Check sheet for the modelled part. Datum: model origin and axes. Units: mm. Give positions to 0.01 mm unless a question says otherwise; leave off trailing zeros. Loops run counter-clockwise (first coordinate to the right, second up) from the corner with the lowest first, then second, coordinate; pieces in that order, holes last. Notation, with made-up numbers: (20, 76.5) - (77, 76.5) arc R30 cw to (77, 101.5) - close; hole circle Ø3 at (59.5, 38.5). An arc over 180 degrees is marked (long way). Use one line per item in the form item = value.
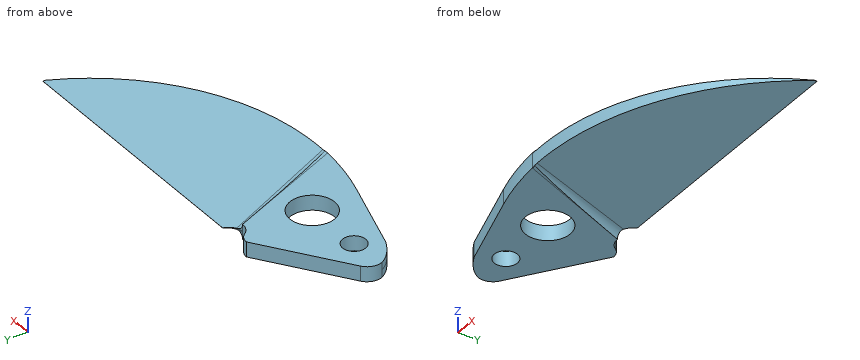
from build123d import *

# Parameters (mm, degrees)
SCHIZZO1_R                   = 3
ESTRUSIONE_ESTRUSIONE1_DEPTH = 1
ESTRUSIONE_ESTRUSIONE2_DEPTH = 0.95
SMUSSO1_SIZE                 = 18
SMUSSO1_SIZE_2               = 0.943340027
SMUSSO2_SIZE                 = 18
SMUSSO2_SIZE_2               = 0.943340027
RACCORDO1_R                  = 0.9
RACCORDO2_R                  = 0.9
TAGLIO_ESTRUSIONE1_DEPTH     = 10
RACCORDO3_R                  = 2
SCHIZZO3_R                   = 1.55
TAGLIO_ESTRUSIONE2_DEPTH     = 41.278810137


with BuildPart() as part:
    # Schizzo1 → Estrusione-Estrusione1 (new, symmetric)
    with BuildSketch(Plane.XY):
        with BuildLine():
            Line((-0.88, 9.5), (-19.130944839, 9.5))
            ThreePointArc((-19.130944839, 9.5), (-20.501263026, 8.610104965), (-20.245662077, 6.99630409))
            Line((-20.245662077, 6.99630409), (-15.960328698, 2.236959209))
            Line((-15.960328698, 2.236959209), (-14.839064722, 1.115695234))
            ThreePointArc((-14.839064722, 1.115695234), (-14.577677448, 0.895591951), (-14.282636649, 0.723197957))
            ThreePointArc((-14.282636649, 0.723197957), (-13.491665822, 0.254040408), (-12.8, -0.352047083))
            add(Edge.make_bspline(
                [(-9.8, -3.018897494), (-12.016366306, -1.919392636), (-12.8, -0.352047083)],
                knots=[0, 0, 0, 0.799118898, 0.799118898, 0.799118898], degree=2))
            Line((-9.8, -3.018897494), (0.594713885, -6.396344771))
            ThreePointArc((0.594713885, -6.396344771), (4.37641373, -7.379985604), (8.248348818, -7.906219091))
            Line((8.248348818, -7.906219091), (2.2, 7.850268275))
            ThreePointArc((2.2, 7.850268275), (1.255676497, 8.087244418), (0.535135135, 8.742015153))
            ThreePointArc((0.535135135, 8.742015153), (-0.077325022, 9.298570279), (-0.88, 9.5))
        make_face()
        Circle(SCHIZZO1_R, mode=Mode.SUBTRACT)
    extrude(amount=ESTRUSIONE_ESTRUSIONE1_DEPTH, both=True)

    # Schizzo1<4> → Estrusione-Estrusione2 (add, symmetric)
    with BuildSketch(Plane.XY):
        with BuildLine():
            ThreePointArc((4.091335816, 9.2), (3.361779551, 8.222303818), (2.2, 7.850268275))
            Line((2.2, 7.850268275), (8.248348818, -7.906219091))
            ThreePointArc((8.248348818, -7.906219091), (26.021901415, -4.20199667), (39.091335816, 8.4))
            Line((39.091335816, 8.4), (39.091335816, 8.7))
            Line((39.091335816, 8.7), (4.091335816, 9.2))
        make_face()
    extrude(amount=ESTRUSIONE_ESTRUSIONE2_DEPTH, both=True)

    # Smusso1
    # the kernel refuses this chamfer: 18, 0.943340027 mm, written as the material it takes off along each edge
    with BuildSketch(Plane(origin=(85.88418926, 8.031530665, 0.95), x_dir=(-0.01428422784103612, -0.9998959488725246, 0.002013023422382226), z_dir=(-0.99989797479951, 0.014284256782850195, 0))) as smusso1_piece_1_section:
        Polygon((SMUSSO1_SIZE * 0.999997973866, -SMUSSO1_SIZE * 0.00201302342238), (-SMUSSO1_SIZE_2 * 0.00201302342258, -SMUSSO1_SIZE_2 * 0.999997973967), (0, 0), align=None)
    smusso1_piece_1 = extrude(amount=128.598827208, mode=Mode.PRIVATE)
    smusso1_piece_1 = split(smusso1_piece_1, bisect_by=Plane(origin=(5.771356931, -1.453434613, 0.613202149), z_dir=(0.9335804264972009, 0.3583679495453028, 0)), keep=Keep.TOP, mode=Mode.PRIVATE)
    add(smusso1_piece_1, mode=Mode.SUBTRACT)

    # Smusso2
    # the kernel refuses this chamfer: 18, 0.943340027 mm, written as the material it takes off along each edge
    with BuildSketch(Plane(origin=(85.88418926, 8.031530665, -0.95), x_dir=(-0.01428422784103612, -0.9998959488725246, -0.002013023422382226), z_dir=(-0.99989797479951, 0.014284256782850195, 0))) as smusso2_piece_1_section:
        Polygon((SMUSSO2_SIZE * 0.999997973866, SMUSSO2_SIZE * 0.00201302342238), (-SMUSSO2_SIZE_2 * 0.00201302342258, SMUSSO2_SIZE_2 * 0.999997973967), (0, 0), align=None)
    smusso2_piece_1 = extrude(amount=128.598827208, mode=Mode.PRIVATE)
    smusso2_piece_1 = split(smusso2_piece_1, bisect_by=Plane(origin=(5.771356931, -1.453434613, -0.613202149), z_dir=(0.9335804264972009, 0.3583679495453028, 0)), keep=Keep.TOP, mode=Mode.PRIVATE)
    add(smusso2_piece_1, mode=Mode.SUBTRACT)

    # Raccordo1
    # the kernel refuses this fillet: 0.9 mm, written as the material it adds along each edge
    with BuildSketch(Plane(origin=(1.410141131, 9.907920978, -0.028429649), x_dir=(-0.017415293659521727, 0.04536839107084769, 0.9988185103603132), z_dir=(0.35794454152552274, -0.9324774108955555, 0.048596124964905896))) as raccordo1_piece_1_section:
        with BuildLine():
            CenterArc((RACCORDO1_R * 0.980734011967, -RACCORDO1_R), RACCORDO1_R, 90, 88.885438442)
            Line((-RACCORDO1_R * 0.0190767888902, -RACCORDO1_R * 0.980548457933), (0, 0))
            Line((0, 0), (RACCORDO1_R * 0.980734011967, 0))
        make_face()
    raccordo1_piece_1 = extrude(amount=21.310749772, mode=Mode.PRIVATE)
    raccordo1_piece_1 = raccordo1_piece_1 & Plane(origin=(10.715020451, 24.750756137, 0.600477284), x_dir=(-0.30901699437494573, -0.9510565162951542, 0), z_dir=(0, 0, 1)) * Cylinder(32.75, 47, mode=Mode.PRIVATE)
    raccordo1_piece_1 = split(raccordo1_piece_1, bisect_by=Plane(origin=(5.151176086, 0.789201867, 1), z_dir=(0, 0, -1)), keep=Keep.TOP, mode=Mode.PRIVATE)
    raccordo1_piece_1 = raccordo1_piece_1 - Plane(origin=(2.2, 9.850268275, 0.600477284), x_dir=(0, -1, 0), z_dir=(0, 0, 1)) * Cylinder(2, 47, mode=Mode.PRIVATE)
    add(raccordo1_piece_1)

    # Raccordo2
    # the kernel refuses this fillet: 0.9 mm, written as the material it adds along each edge
    with BuildSketch(Plane(origin=(1.410141131, 9.907920978, 0.028429649), x_dir=(-0.017415293659511128, 0.04536839107085176, -0.9988185103603133), z_dir=(0.35794454152552274, -0.9324774108955555, -0.048596124964905896))) as raccordo2_piece_1_section:
        with BuildLine():
            CenterArc((RACCORDO2_R * 0.980734011967, RACCORDO2_R), RACCORDO2_R, 181.114561558, 88.885438442)
            Line((-RACCORDO2_R * 0.0190767888902, RACCORDO2_R * 0.980548457933), (0, 0))
            Line((0, 0), (RACCORDO2_R * 0.980734011967, 0))
        make_face()
    raccordo2_piece_1 = extrude(amount=21.310749772, mode=Mode.PRIVATE)
    raccordo2_piece_1 = split(raccordo2_piece_1, bisect_by=Plane(origin=(5.151178194, 0.789195879, -1), z_dir=(0, 0, 1)), keep=Keep.TOP, mode=Mode.PRIVATE)
    raccordo2_piece_1 = raccordo2_piece_1 & Plane(origin=(10.715020451, 24.750756137, -0.600477223), x_dir=(-0.3090169943750401, -0.9510565162951234, 0), z_dir=(0, 0, 1)) * Cylinder(32.75, 47, mode=Mode.PRIVATE)
    raccordo2_piece_1 = raccordo2_piece_1 - Plane(origin=(2.2, 9.850268275, -0.600477223), x_dir=(0, -1, 0), z_dir=(0, 0, 1)) * Cylinder(2, 47, mode=Mode.PRIVATE)
    add(raccordo2_piece_1)

    # Schizzo2 → Taglio-Estrusione1 (cut)
    with BuildSketch(Plane.XY.offset(1)):
        Polygon((-0.88, 9.5), (-30.88, -10.735255505), (-30.88, 9.5), align=None)
    extrude(amount=-TAGLIO_ESTRUSIONE1_DEPTH, mode=Mode.SUBTRACT)

    # Raccordo3
    # the kernel refuses this fillet: 2 mm, written as the material it takes off along each edge
    with BuildSketch(Plane(origin=(-14.059482684, 0.610326682, -7.107620692), x_dir=(0.7945891525397701, -0.6071474933375991, 0), z_dir=(0, 0, 1))) as raccordo3_piece_1:
        with BuildLine():
            CenterArc((2.675251835, 1.676756542), RACCORDO3_R, 161.383532721, 75.585730468)
            Line((0.779898436, 2.315219927), (0.741991368, 2.327989195))
            Line((0.741991368, 2.327989195), (-0.037907068, 0.012769268))
            Line((-0.037907068, 0.012769268), (0.006340296, -0.039494312))
            ThreePointArc((0.006340296, -0.039494312), (0.792537049, 0.023211061), (1.563270543, -0.033535131))
            Line((1.563270543, -0.033535131), (1.585074098, 0))
        make_face()
    extrude(amount=14.215241383, mode=Mode.SUBTRACT)

    # Schizzo3 → Taglio-Estrusione2 (cut, through all)
    with BuildSketch(Plane(origin=(0, 0, -1), x_dir=(-1, 0, 0), z_dir=(0, 0, -1))):
        with Locations((8, 0)):
            Circle(SCHIZZO3_R)
    extrude(amount=-TAGLIO_ESTRUSIONE2_DEPTH, mode=Mode.SUBTRACT)


solid = part.part
Item 1: Section check A-A on x = 0. Record the boundary of the cut face in (y, z), then the cut area to 3 significant figures.
Answer block:
outline = (-6.2, -1) - (-3, -1) - (-3, 1) - (-6.2, 1) - close; (3, -1) - (9.25, -1) - (9.25, 1) - (3, 1) - close
area = 18.9 mm2
Item 2: Section check B-B on y = 0.5. Give the number of separate pieces and of enclosed holes in the cut face, then the cut area to 3 significant figures.
Answer block:
separate_pieces = 3
enclosed_holes = 0
area = 43.5 mm2
Item 3: Gauge pin test, flat ends, axial feed: P1, Ø10, axis at x = 25.5, y = 7, coming from the +Z side; P2, Ø3, axis at x = -8, y = 0, coming from the +Z side. Record the tip position at first contact, or that the pin passes through.
Answer block:
P1 = 0.37
P2 = through
Item 4: Section check D-D on x = -8. Record the boundary of the cut face in (y, z).
Answer block:
outline = (-3.6, -1) - (-1.55, -1) - (-1.55, 1) - (-3.6, 1) - close; (1.55, -1) - (4.7, -1) - (4.7, 1) - (1.55, 1) - close
Item 5: Thickness scan on L1, parallel to X at y = -2, z = -0.4; L2, parallel to Y at x = -8, z = 0.55; L3, parallel to Y at x = -0.5, z = 0.55. Record the ranges inside material, lowest first.
Answer block:
L1 = -11.42 to -2.24, 2.24 to 29.61
L2 = -3.6 to -1.55, 1.55 to 4.7
L3 = -6.04 to -2.96, 2.96 to 9.46
